Input: part model. Units: mm. Frame: model coordinates. Face numbers are marked on the shaded views. A direction names the side the tool comes from. Give positions to 0.01 mm unless a question says otherwise; leave off trailing zeros. Loops run counter-clockwise (first coordinate to the right, second up) from the corner with the lowest first, then second, coordinate; pieces in that order, holes last. Notation, with made-up numbers: (-1, 42.25) -> (8, 42.25) arc R26 ccw to (8, 56.25) -> close; hole circle Ø8 at (31.25, 45). An arc over 180 degrees is marked (long way). Answer as a JSON object with one key per item and string values.
```python
from build123d import *

# Parameters (mm, degrees)
F1_DEPTH  = 38.1
F3_DEPTH  = 38.101
F5_R      = 25.4
F6_DEPTH  = 50.8
F6_FACE_R = 25.4
F7_DEPTH  = 25.4
F8_R      = 12.7
F9_DEPTH  = 76.201
F11_DEPTH = 50.801


with BuildPart() as f1:
    # F0 (on Right) → F1 (new body)
    with BuildSketch(Plane.YZ):
        Polygon((-38.1, 0), (0, 0), (0, 50.8), (-12.7, 50.8), (-12.7, 38.1), (-38.1, 38.1), align=None)
    extrude(amount=-F1_DEPTH)

    # F2 (on Front) → F3 (cut, through all)
    with BuildSketch(Plane.XZ):
        Polygon((-38.1, 50.8), (0, 0), (0, 50.8), align=None)
    extrude(amount=F3_DEPTH, mode=Mode.SUBTRACT)

    # F5 (on offset) → F6 (join)
    with BuildSketch(Plane.YZ.offset(12.7)):
        with Locations((-25.4, 0)):
            Circle(F5_R)
    extrude(amount=-F6_DEPTH)

    # F6_face (on face) → F7 (join)
    with BuildSketch(Plane(origin=(12.7, -25.4, 0), x_dir=(0, 1, 0), z_dir=(1, 0, 0))):
        Circle(F6_FACE_R)
    extrude(amount=F7_DEPTH)

    # F8 (on face) → F9 (cut, through all)
    with BuildSketch(Plane.YZ.offset(38.1)):
        with Locations((-25.4, 0)):
            Circle(F8_R)
    extrude(amount=-F9_DEPTH, mode=Mode.SUBTRACT)

    # F10 (on Front) → F11 (cut, through all)
    with BuildSketch(Plane.XZ):
        Polygon((38.1, 9.525), (38.1, 25.4), (12.7, 25.4), (12.7, 0), (12.7, -9.525), (25.4, -9.525), (25.4, 9.525), align=None)
    extrude(amount=F11_DEPTH, mode=Mode.SUBTRACT)


solid = f1.part
```
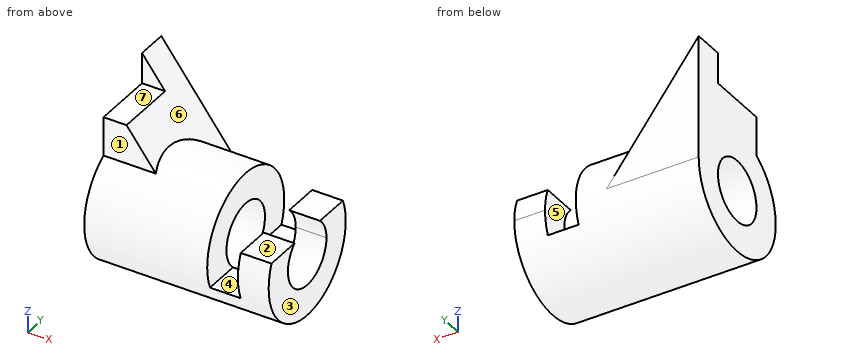
Q1. Section B-B, the plane y = -35. Return the cut outline in (x, z) (3 decimals), then the cut area to 3 significant figures.
Evaluation:
{"outline": "(-38.1, -23.516) -> (38.1, -23.516) -> (38.1, -8.314) -> (25.4, -8.314) -> (25.4, -9.525) -> (12.7, -9.525) -> (12.7, -8.314) -> (-38.1, -8.314) -> close; (-38.1, 8.314) -> (12.7, 8.314) -> (12.7, 23.516) -> (-17.637, 23.516) -> (-28.575, 38.1) -> (-38.1, 38.1) -> close; (25.4, 8.314) -> (38.1, 8.314) -> (38.1, 9.525) -> (25.4, 9.525) -> close", "area": "2,150 mm2"}
Q2. Section C-C, the plane z = 3. Return the cut outline in (x, y).
Evaluation:
{"outline": "(-38.1, -50.62) -> (12.7, -50.62) -> (12.7, -37.74) -> (-38.1, -37.74) -> close; (-38.1, -13.06) -> (12.7, -13.06) -> (12.7, -0.18) -> (-2.25, -0.18) -> (-2.25, 0) -> (-38.1, 0) -> close; (25.4, -50.62) -> (38.1, -50.62) -> (38.1, -37.74) -> (25.4, -37.74) -> close; (25.4, -13.06) -> (38.1, -13.06) -> (38.1, -0.18) -> (25.4, -0.18) -> close"}
Q3. Access query for the marked faces 1, 2, 3 and 4. Directions: +Z, -Z, +X, -X, +Y, -Y. A direction counts if a zero-diameter tool reaches every point of the face in a straight line with its end or side. Return the directions, or none.
Evaluation:
{"face 1": "+Z, +X, -X, -Y", "face 2": "+Z, +X, +Y, -Y", "face 3": "+Z, -Z, +X, +Y, -Y", "face 4": "+Z, +Y, -Y"}
Q4. Pin query (flat end, axial travel): pin 1 (8 mm diameter, centred on x = -23.5, z = 33.5, fed in from -Y); pin 2 (6.5 mm diameter, centred on x = 20, y = -11, fed in from +Z) (3 decimals); pin 3 (7.5 mm diameter, centred on x = -35.5, z = 43.5, fed in from -Y); pin 4 (5 mm diameter, centred on x = 17.5, z = 4, fed in from +Y). Return the tip coordinate at first contact, or that it passes through.
Evaluation:
{"pin 1": "stops at y = -38.1", "pin 2": "stops at z = -9.525", "pin 3": "stops at y = -12.7", "pin 4": "passes through"}
Q5. Ray query, line 1 along Y through (x, z) = (-3, 0); line 2 along Z through (x, y) = (-16, -25.4); line 3 along X through (y, z) = (-20, 13.5). Return the intervals inside material, ascending.
Evaluation:
{"line 1": "y = -50.8 to -38.1, -12.7 to 0", "line 2": "z = -25.4 to -12.7, 12.7 to 25.4", "line 3": "x = -38.1 to 12.7"}
Q6. Section A-A, the plane y = -25.4. Return the cut outline in (x, z) (3 decimals).
Evaluation:
{"outline": "(-38.1, -25.4) -> (38.1, -25.4) -> (38.1, -12.7) -> (-38.1, -12.7) -> close; (-38.1, 12.7) -> (12.7, 12.7) -> (12.7, 25.4) -> (-19.05, 25.4) -> (-28.575, 38.1) -> (-38.1, 38.1) -> close"}
Q7. Draft query along X for the marked faces 5, 6 and 7. Return one class per face: +X half, -X half, draft (parallel to the pull), parting line (faces both ways), or undercut.
Evaluation:
{"face 5": "undercut", "face 6": "+X half", "face 7": "draft"}
Q8. Section D-D, the plane x = 26.5. Return the cut outline in (y, z) (3 decimals), then the cut area to 3 significant figures.
Evaluation:
{"outline": "(-48.946, 9.525) arc R25.4 ccw (long way) to (-1.854, 9.525) -> (-17, 9.525) arc R12.7 cw (long way) to (-33.8, 9.525) -> close", "area": "1,020 mm2"}
